Part model, mm, in its own coordinate system. A direction names the side the tool comes from. Round coordinates to 2 decimals unless told otherwise and drop trailing zeros. Loops run counter-clockwise (first coordinate to the right, second up) from the corner with the lowest first, then second, coordinate; pieces in that order, holes last. Notation, with made-up numbers: (87.25, 49) -> (119.25, 49) arc R25 cw to (119.25, 71) -> close; hole circle Ø8 at (50.25, 23.5). An arc over 180 degrees is marked (long way). Answer as CSV lines item,"result".
from build123d import *

# Parameters (mm, degrees)
ESQUISSE1_W             = 330
ESQUISSE1_H             = 75
BOSS_EXTRU_1_DEPTH      = 6
ESQUISSE2_W             = 134
ESQUISSE2_H             = 6
ESQUISSE2_W_2           = 6
ESQUISSE2_H_2           = 19
ESQUISSE2_H_3           = 29
ENL_V_MAT_EXTRU_1_DEPTH = 6
ESQUISSE3_W             = 50
ESQUISSE3_H             = 6
BOSS_EXTRU_2_DEPTH      = 70
ESQUISSE5_W             = 6
ESQUISSE5_H             = 40
BOSS_EXTRU_3_DEPTH      = 6
ESQUISSE6_W             = 268
ESQUISSE6_H             = 6
BOSS_EXTRU_4_DEPTH      = 20
ESQUISSE7_W             = 58.270575025
ESQUISSE7_H             = 148.089415769
ESQUISSE7_W_2           = 60
ESQUISSE7_H_2           = 6
ENL_V_MAT_EXTRU_3_DEPTH = 361.50104022
ESQUISSE8_W             = 6
ESQUISSE8_H             = 29.5
BOSS_EXTRU_5_DEPTH      = 6


with BuildPart() as part:
    # Esquisse1 → Boss.-Extru.1 (new body)
    with BuildSketch(Plane.XY):
        with Locations((-165, 37.5)):
            Rectangle(ESQUISSE1_W, ESQUISSE1_H)
    extrude(amount=BOSS_EXTRU_1_DEPTH)

    # Esquisse2 → Enlèv. mat.-Extru.1 (cut)
    with BuildSketch(Plane.XY.offset(6)):
        Polygon((-330, 0), (-270, 0), (-270, 6), (-324, 6), (-324, 36), (-330, 36), align=None)
        Polygon((0, 0), (-60, 0), (-60, 6), (-6, 6), (-6, 26), (0, 26), align=None)
        with Locations((-165, 3)):
            Rectangle(ESQUISSE2_W, ESQUISSE2_H)
        with Locations((-327, 65.5)):
            Rectangle(ESQUISSE2_W_2, ESQUISSE2_H_2)
        with Locations((-3, 60.5)):
            Rectangle(ESQUISSE2_W_2, ESQUISSE2_H_3)
    extrude(amount=-ENL_V_MAT_EXTRU_1_DEPTH, mode=Mode.SUBTRACT)

    # Esquisse3 → Boss.-Extru.2 (add)
    with BuildSketch(Plane(origin=(0, 75, 0), x_dir=(1, 0, 0), z_dir=(0, 1, 0))):
        with Locations((-31, -3)):
            Rectangle(ESQUISSE3_W, ESQUISSE3_H)
    extrude(amount=BOSS_EXTRU_2_DEPTH)

    # Esquisse5 → Boss.-Extru.3 (add)
    with BuildSketch(Plane(origin=(-6, 0, 0), x_dir=(0, 0, -1), z_dir=(1, 0, 0))):
        with Locations((-3, 105)):
            Rectangle(ESQUISSE5_W, ESQUISSE5_H)
    extrude(amount=BOSS_EXTRU_3_DEPTH)

    # Esquisse6 → Boss.-Extru.4 (add)
    with BuildSketch(Plane(origin=(0, 75, 0), x_dir=(1, 0, 0), z_dir=(0, 1, 0))):
        with Locations((-190, -3)):
            Rectangle(ESQUISSE6_W, ESQUISSE6_H)
    extrude(amount=BOSS_EXTRU_4_DEPTH)

    # Esquisse7 → Enlèv. mat.-Extru.3 (cut, through all)
    with BuildSketch(Plane.XY.offset(6)):
        with Locations((-26.864712488, 70.955292116)):
            Rectangle(ESQUISSE7_W, ESQUISSE7_H)
        with Locations((-136, 92)):
            Rectangle(ESQUISSE7_W_2, ESQUISSE7_H_2)
        with Locations((-244, 92)):
            Rectangle(ESQUISSE7_W_2, ESQUISSE7_H_2)
    extrude(amount=-ENL_V_MAT_EXTRU_3_DEPTH, mode=Mode.SUBTRACT)

    # Esquisse8 → Boss.-Extru.5 (add)
    with BuildSketch(Plane(origin=(-56, 0, 0), x_dir=(0, 0, -1), z_dir=(1, 0, 0))):
        with Locations((-3, 20.75)):
            Rectangle(ESQUISSE8_W, ESQUISSE8_H)
        with Locations((-3, 80.25)):
            Rectangle(ESQUISSE8_W, ESQUISSE8_H)
    extrude(amount=BOSS_EXTRU_5_DEPTH)


solid = part.part
Q1. Saw through at A-A, the plane z = 2.55. Write the cut outline in (x, y), then the cut area to 3 significant figures.
Geometry results:
outline,"(-330, 36) -> (-324, 36) -> (-324, 6) -> (-270, 6) -> (-270, 0) -> (-232, 0) -> (-232, 6) -> (-98, 6) -> (-98, 0) -> (-60, 0) -> (-60, 6) -> (-50, 6) -> (-50, 35.5) -> (-56, 35.5) -> (-56, 65.5) -> (-50, 65.5) -> (-50, 95) -> (-106, 95) -> (-106, 89) -> (-166, 89) -> (-166, 95) -> (-214, 95) -> (-214, 89) -> (-274, 89) -> (-274, 95) -> (-324, 95) -> (-324, 56) -> (-330, 56) -> close"
area,"24,100 mm2"
Q2. Two-plate mould, pull along X, no slides. Class faces 1 (the face through (-324, 21, 3)), 2 (the face through (-136, 89, 3)), 3 (the face through (-60, 3, 3)): pulls with the +X half, pulls with the -X half, needs draft (parallel to the pull), parting line crosses it, or undercut.
Geometry results:
face 1,"pulls with the -X half"
face 2,"undercut"
face 3,"pulls with the +X half"
Q3. Saw through at B-B, the plane x = -155.5. Write the cut outline in (y, z).
Geometry results:
outline,"(6, 0) -> (89, 0) -> (89, 6) -> (6, 6) -> close"
Q4. Saw through at C-C, the plane y = 20.5. Write the cut outline in (x, z), then the cut area to 3 significant figures.
Geometry results:
outline,"(-324, 0) -> (-50, 0) -> (-50, 6) -> (-324, 6) -> close"
area,"1,640 mm2"
Q5. Drill centre lines: line 1 along X through (y, z) = (18.5, 2.55); line 2 along Y through (x, z) = (-316, 3); line 3 along Y through (x, z) = (-268, 1.1). Where is each one in solid material? Low to high.
Geometry results:
line 1,"-324 to -50"
line 2,"6 to 95"
line 3,"0 to 89"
Q6. Which spindle directions (+Z, -Z, +X, -X, +Y, -Y) get a long thin tool onto all of the face, cutting with end or side? Do faces 4 (the face through (-53, 35.5, 3)), 5 (the face through (-274, 92, 3)), 6 (the face through (-327, 56, 3)), 7 (the face through (-327, 36, 3)). Say none if no direction does.
Geometry results:
face 4,"+Z, -Z, +X"
face 5,"+Z, -Z, +Y"
face 6,"+Z, -Z, -X, +Y"
face 7,"+Z, -Z, -X, -Y"
Q7. Drop flat-ended pins along their axis: P1, Ø3, axis at x = -327.5, z = 2, coming from the -Y side; P2, Ø2, axis at y = 31, z = 2, coming from the -X side; P3, Ø1.8, axis at y = 3, z = 4, coming from the +X side. Give the stop position or say it passes through.
Geometry results:
P1,"y = 36"
P2,"x = -324"
P3,"x = -60"
